```python
from build123d import *

# Parameters (mm, degrees)
F0_W     = 150.236324
F0_H     = 81.752524
F1_DEPTH = 50
F3_DEPTH = 166
F5_DEPTH = 10
F7_R     = 12.648051
F7_R_2   = 12.64805
F8_DEPTH = 89.9


with BuildPart() as f1:
    # F0 (on Front) → F1 (new body)
    with BuildSketch(Plane.XZ):
        Rectangle(F0_W, F0_H)
    extrude(amount=F1_DEPTH)

    # F2 (on face) → F3 (cut)
    with BuildSketch(Plane.XZ.offset(50)):
        with BuildLine():
            Line((20.626348, 40.876262), (-20.883331, 40.876262))
            ThreePointArc((-20.883331, 40.876262), (-0.128492, 23.526994), (20.626348, 40.876262))
        make_face()
    extrude(amount=-F3_DEPTH, mode=Mode.SUBTRACT)

    # F4 (on face) → F5 (join)
    with BuildSketch(Plane.XZ.offset(50)):
        with BuildLine():
            ThreePointArc((20.626348, 40.876262), (-0.128492, 23.527007), (-20.883331, 40.876262))
            Line((-20.883331, 40.876262), (-31.085527, 40.876262))
            ThreePointArc((-31.085527, 40.876262), (-0.12849, 13.638671), (30.828548, 40.876262))
            Line((30.828548, 40.876262), (20.626348, 40.876262))
        make_face()
    extrude(amount=F5_DEPTH)

    # F6: F1 across face


with BuildPart() as f1_1:
    add(f1.part)
    add(f1.part.mirror(Plane(origin=(0.005929, 0, -1.550904), x_dir=(1, 0, 0), z_dir=(0, 1, 0))))

    # F7 (on face) → F8 (cut)
    with BuildSketch(Plane.XY.offset(40.876262)):
        with Locations((-47.940791, 0)):
            Circle(F7_R)
        with Locations((47.94079, 0)):
            Circle(F7_R_2)
    extrude(amount=-F8_DEPTH, mode=Mode.SUBTRACT)


solid = f1_1.part
```
Model file for the job. Use its own axes, mm. A direction names the side the tool comes from. Coordinates: 2 decimals unless noted, no trailing zeros. Loops run counter-clockwise (first coordinate to the right, second up) from the corner with the lowest first, then second, coordinate; pieces in that order, holes last. Notation, with made-up numbers: M 71.25,52 L 119.25,52 A15 ccw 119.25,58 Z; hole C 15.25,-36.5 d10. An arc over 180 degrees is marked long. Use CSV: the item, a comma, the result in double quotes. Start each with the question number.
1. Band-saw the part on B-B, the plane z = 21. List the corners of the cut face in (x, y), then the cut area to 3 significant figures.
2. Two-plate mould, pull along Y, no slides. Class faces 1 (the cylindrical face through (0.28, -54.93, 23.53)), 2 (the cylindrical face through (60.005, 3.799, 0.572)), 3 (the flat face through (-1, 60, 21)): pulls with the +Y half, pulls with the -Y half, needs draft (parallel to the pull), parting line crosses it, or undercut.
3. Band-saw the part on C-C, the plane x = 37. List the corners of the cut face in (y, z), then the cut area to 3 significant figures.
4. Tool access for faces 4 (the flat face through (-1, -50, 1)), 5 (the cylindrical face through (-0.759, 54.93, 13.645)), 6 (the flat face through (75.118, -1, -1)): list every direction of +Z, -Z, +X, -X, +Y, -Y with a clear straight run to the whole face (end or side of a thin tool).
5. Band-saw the part on D-D, the plane y = 48. List the corners of the cut face in (x, z), then the cut area to 3 significant figures.
6. Flat gauge pins, fed straight in: pin 1 (12 mm diameter, centred on x = -30.5, z = 21, fed in from +Y); pin 2 (12 mm diameter, centred on x = -23.5, z = -3.5, fed in from -Y); pin 3 (1.5 mm diameter, centred on x = 1.5, y = 36.5, fed in from +Z). Where does each tip first touch, or does it go through?
7. Band-saw the part on A-A, the plane y = 0. List the corners of the cut face in (x, z).
8. Probe probe 1 along X at (y, z) = (11, 19.5); probe 2 along X at (y, z) = (-2, 13); probe 3 along X at (y, z) = (-46, 34). List the from-to ranges inside material, lowest first. Write a range as [from, to].
Entries:
1,outline,"M -75.12,-50 L -20.26,-50 L -20.26,-60 L 20,-60 L 20,-50 L 75.12,-50 L 75.12,50 L 20,50 L 20,60 L -20.26,60 L -20.26,50 L -75.12,50 Z; hole C -47.94,0 d25.3; hole C 47.94,0 d25.3"
1,area,"14,800 mm2"
2,face 1,"needs draft"
2,face 2,"undercut"
2,face 3,"pulls with the +Y half"
3,outline,"M -50,-40.88 L -6.35,-40.88 L -6.35,40.88 L -50,40.88 Z; M 6.35,-40.88 L 50,-40.88 L 50,40.88 L 6.35,40.88 Z"
3,area,"7,140 mm2"
4,face 4,"-Z, -Y"
4,face 5,"-Z, +Y"
4,face 6,"+Z, -Z, +X, +Y, -Y"
5,outline,"M -75.12,-40.88 L 75.12,-40.88 L 75.12,40.88 L 20.63,40.88 A21.09 cw -20.88,40.88 L -75.12,40.88 Z"
5,area,"11,700 mm2"
6,pin 1,"stops at y = 50"
6,pin 2,"stops at y = -50"
6,pin 3,"stops at z = 23.66"
7,outline,"M -75.12,-40.88 L -60.59,-40.88 L -60.59,40.88 L -75.12,40.88 Z; M -35.29,-40.88 L 35.29,-40.88 L 35.29,40.88 L 20.63,40.88 A21.09 cw -20.88,40.88 L -35.29,40.88 Z; M 60.59,-40.88 L 75.12,-40.88 L 75.12,40.88 L 60.59,40.88 Z"
8,probe 1,"x = [-75.12, -54.18], [-41.7, 41.7], [54.18, 75.12]"
8,probe 2,"x = [-75.12, -60.43], [-35.45, 35.45], [60.43, 75.12]"
8,probe 3,"x = [-75.12, -18.35], [18.09, 75.12]"
